Build history of the part. All positions in model axes, mm. Round coordinates to 2 decimals unless told otherwise and drop trailing zeros. Loops run counter-clockwise (first coordinate to the right, second up) from the corner with the lowest first, then second, coordinate; pieces in that order, holes last.
from build123d import *

# Parameters (mm, degrees)
SKETCH2_R   = 6.604
SKETCH2_R_2 = 5.334


with BuildPart() as part:
    # Sweep-Thin1: sweep along a path in Sketch1
    with BuildLine(Plane(origin=(0, 0, 0), x_dir=(0, 0, -1), z_dir=(1, 0, 0))) as sweep_thin1_path:
        Line((0, 0), (0, 19.05))
        ThreePointArc((0, 19.05), (-5.579615818, 32.520384182), (-19.05, 38.1))
        Line((-19.05, 38.1), (-38.1, 38.1))
    # Sketch2 → Sweep-Thin1 (sweep)
    with BuildSketch(Plane(origin=(0, 0, 0), x_dir=(1, 0, 0), z_dir=(0, 1, 0))):
        Circle(SKETCH2_R)
        Circle(SKETCH2_R_2, mode=Mode.SUBTRACT)
    sweep(path=sweep_thin1_path.line)


solid = part.part
(1) Probe line 1 (X direction, y = 8, z = 0); line 2 (Y direction, x = 0, z = 34.25). List the from-to ranges inside material, lowest first.
Responses:
line 1: x = -6.6 to -5.33, 5.33 to 6.6
line 2: y = 31.5 to 32.77, 43.43 to 44.7
(2) Slice it at D-D on y = 11. List the corners of the cut face in (x, z).
Responses:
outline: circle Ø13.21 at (0, 0); hole circle Ø10.67 at (0, 0)
(3) Pull direction Y, two halves, no side cores. Call faces 1 (the face through (-1.432, 31.653, 28.708)), 2 (the face through (0, 44, 38.1)), 3 (the face through (-1.156, 32.893, 28.708)): +Y half, -Y half, draft (parallel to the pull), parting line (faces both ways), or undercut.
Responses:
face 1: parting line
face 2: draft
face 3: undercut
(4) Slice it at A-A on x = 0. List the corners of the cut face in (y, z), plus the area to 3 significant figures.
Responses:
outline: (0, -6.6) - (19.05, -6.6) arc R25.65 ccw to (44.7, 19.05) - (44.7, 38.1) - (43.43, 38.1) - (43.43, 19.05) arc R24.38 cw to (19.05, -5.33) - (0, -5.33) - close; (0, 5.33) - (19.05, 5.33) arc R13.72 ccw to (32.77, 19.05) - (32.77, 38.1) - (31.5, 38.1) - (31.5, 19.05) arc R12.45 cw to (19.05, 6.6) - (0, 6.6) - close
area: 173 mm2
(5) Slice it at B-B on z = 28.5. List the corners of the cut face in (x, y), plus the area to 3 significant figures.
Responses:
outline: circle Ø13.21 at (0, 38.1); hole circle Ø10.67 at (0, 38.1)
area: 47.6 mm2
(6) Pin check, flat tips, straight feed: P1, Ø6, axis at y = 23.5, z = 12.5, coming from the +X side; P2, Ø6.5, axis at x = 0, z = 0, coming from the +Y side; P3, Ø5, axis at x = 2.5, y = 13.5, coming from the +Z side; P4, Ø1, axis at x = -1.5, y = 26.5, coming from the -Z side. Stop position of each tip, or through.
Responses:
P1: passes through
P2: stops at y = 39.26
P3: stops at z = 6.6
P4: stops at z = -5.5
(7) Slice it at C-C on x = -4.25. List the corners of the cut face in (y, z).
Responses:
outline: (0, -5.05) - (19.05, -5.05) arc R24.1 ccw to (43.15, 19.05) - (43.15, 38.1) - (41.32, 38.1) - (41.32, 19.05) arc R22.27 cw to (19.05, -3.22) - (0, -3.22) - close; (0, 3.22) - (19.05, 3.22) arc R15.83 ccw to (34.88, 19.05) - (34.88, 38.1) - (33.05, 38.1) - (33.05, 19.05) arc R14 cw to (19.05, 5.05) - (0, 5.05) - close
